Geometry: see drawing. Coordinates: mm, zero at the bounding-box minimum. Round coordinates to 2 decimals unless told otherwise and drop trailing zeros. Order: outer loops, then holes, each group sorted by start corner. A loop starts at its lowest first (then second) coordinate and runs counter-clockwise, first axis right, second up.
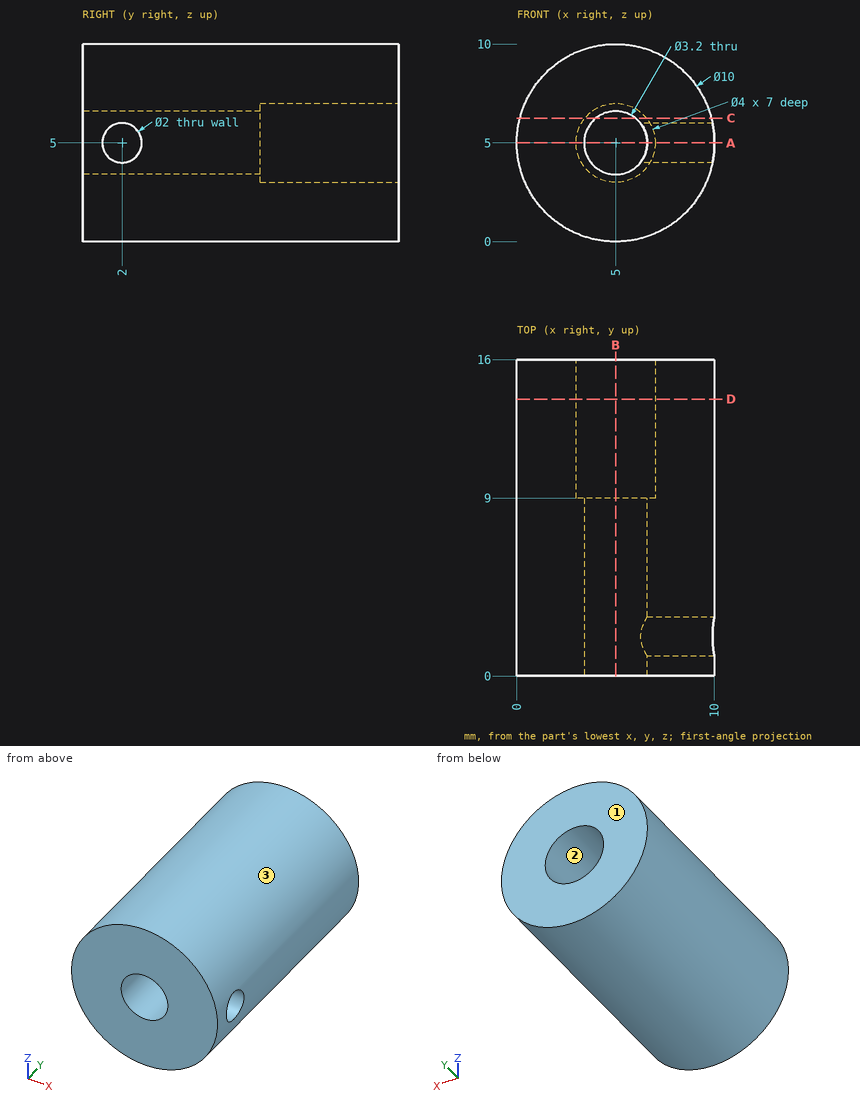
1. Section A-A on z = 5. Return loops of the section in (x, y).
2. First-contact query: pin 1 (3 mm diameter, centred on y = 10.5, z = 7.5, fed in from +X); pin 2 (2.5 mm diameter, centred on x = 5, z = 5, fed in from -Y); pin 3 (3 mm diameter, centred on y = 3.5, z = 1, fed in from +X); pin 4 (5 mm diameter, centred on x = 1, y = 5.5, fed in from +Z). Flat tips, straight axial feed; report the tip coordinate or a pass-through.
3. Line query: line 1 along Z through (x, y) = (5, 12.5); line 2 along X through (y, z) = (3.75, 8); line 3 along Z through (x, y) = (5, 6.5). Output: solid intervals per line, ascending.
4. Pull-direction query (Z, two-part tool) for the marked faces 1, 2 and 3; classes: released by +Z, released by -Z, zero draft, split by the parting line, or undercut.
5. Section D-D on y = 14. Return loops of the section in (x, z).
6. Section B-B on x = 5. Return loops of the section in (y, z), plus the area to 3 significant figures.
7. Section C-C on z = 6.25. Return loops of the section in (x, y), plus the area to 3 significant figures.
Result:
1. outline: (0, 0) - (3.4, 0) - (3.4, 9) - (3, 9) - (3, 16) - (0, 16) - close; (6.6, 0) - (10, 0) - (10, 1) - (6.6, 1) - close; (6.6, 3) - (10, 3) - (10, 16) - (7, 16) - (7, 9) - (6.6, 9) - close
2. pin 1: stops at x = 9.9
2. pin 2: passes through
2. pin 3: stops at x = 9.33
2. pin 4: stops at z = 9.77
3. line 1: z = 0 to 3, 7 to 10
3. line 2: x = 1 to 9
3. line 3: z = 0 to 3.4, 6.6 to 10
4. face 1: zero draft
4. face 2: undercut
4. face 3: split by the parting line
5. outline: circle Ø10 at (5, 5); hole circle Ø4 at (5, 5)
6. outline: (0, 0) - (16, 0) - (16, 3) - (9, 3) - (9, 3.4) - (0, 3.4) - close; (0, 6.6) - (9, 6.6) - (9, 7) - (16, 7) - (16, 10) - (0, 10) - close
6. area: 103 mm2
7. outline: (0.16, 0) - (4, 0) - (4, 9) - (3.44, 9) - (3.44, 16) - (0.16, 16) - close; (6, 0) - (9.84, 0) - (9.84, 16) - (6.56, 16) - (6.56, 9) - (6, 9) - close
7. area: 115 mm2
